Here's how the part is built. I have some questions about the finished solid (model axes, mm). A direction names the side the tool comes from. Round coordinates to 2 decimals unless told otherwise and drop trailing zeros. Write each loop counter-clockwise with the first axis right and the second up, starting at its lowest first coordinate (ties: lowest second). Pieces come first, ordered by that corner, then holes. Notation, with made-up numbers: (17.5, 60) -> (34.5, 60) arc R22 ccw to (34.5, 82) -> close; hole circle Ø2 at (-18.5, 40.25). An arc over 180 degrees is marked (long way). Put each result on its own line as item: value. Start each with the question number.
1) I want a section at A-A, the plane z = -1.75. List the corners of the cut face in (x, y) for me.
2) If I drill on line 1 along Y through (x, z) = (0, -1.95); line 2 along Y through (x, z) = (21, 1.7); line 3 along X through (y, z) = (-15.5, 1.85), over which ranges is the centre line in solid material (lowest first)? Write a range as [from, to].
3) We'd pull the mould along X, two halves only. Please class faces 5 (the flat face through (14.75, 0, 0)), 6 (the cylindrical face through (-18.365, -18.049, 0.042)), 7 (the flat face through (0, 14.75, 0)): released by +X, released by -X, zero draft, split by the parting line, or undercut.
4) Will these pins go through, and if not, where does the flat tip stop? P1, Ø3, axis at y = 18.5, z = 0, coming from the +X side; P2, Ø1.8, axis at y = -19.5, z = -1, coming from the +X side; P3, Ø1.5, axis at x = -12.5, z = -0.5, coming from the -Y side.
5) I want a section at C-C, the plane z = 1.25. List the corners of the cut face in (x, y) for me.
6) Which directions (+Z, -Z, +X, -X, +Y, -Y) give clear straight access to the entire face, cutting with the end or side of a thin tool? Please do faces 1 (the flat face through (-14.75, 0, 0)), 2 (the cylindrical face through (-2.4, -4.5, -1.8)), 3 (the flat face through (4.25, -20, 0)), 4 (the flat face through (-4.25, 20, 0)).
7) I want a section at B-B, the plane y = 17. List the corners of the cut face in (x, z) for me.
8) I want a section at D-D, the plane x = 21.5. List the corners of the cut face in (y, z) for me, then the cut area to 3 significant figures.
from build123d import *

# Parameters (mm, degrees)
BOSS_EXTRUDE1_DEPTH = 3
SKETCH3_R           = 5.1
CUT_EXTRUDE1_DEPTH  = 2.5


with BuildPart() as part:
    # Sketch2 → Boss-Extrude1 (new, symmetric)
    with BuildSketch(Plane.XY):
        with BuildLine():
            Line((-25.396850198, 4.25), (-14.75, 4.25))
            Line((-14.75, 4.25), (-14.75, -4.25))
            Line((-14.75, -4.25), (-25.396850198, -4.25))
            ThreePointArc((-25.396850198, -4.25), (-18.207999616, -18.207999616), (-4.25, -25.396850198))
            Line((-4.25, -25.396850198), (-4.25, -14.75))
            Line((-4.25, -14.75), (4.25, -14.75))
            Line((4.25, -14.75), (4.25, -25.396850198))
            ThreePointArc((4.25, -25.396850198), (18.207999616, -18.207999616), (25.396850198, -4.25))
            Line((25.396850198, -4.25), (14.75, -4.25))
            Line((14.75, -4.25), (14.75, 4.25))
            Line((14.75, 4.25), (25.396850198, 4.25))
            ThreePointArc((25.396850198, 4.25), (18.207999616, 18.207999616), (4.25, 25.396850198))
            Line((4.25, 25.396850198), (4.25, 14.75))
            Line((4.25, 14.75), (-4.25, 14.75))
            Line((-4.25, 14.75), (-4.25, 25.396850198))
            ThreePointArc((-4.25, 25.396850198), (-18.207999616, 18.207999616), (-25.396850198, 4.25))
        make_face()
    extrude(amount=BOSS_EXTRUDE1_DEPTH, both=True)

    # Sketch3 → Cut-Extrude1 (cut)
    with BuildSketch(Plane(origin=(0, 0, -3), x_dir=(-1, 0, 0), z_dir=(0, 0, -1))):
        Circle(SKETCH3_R)
    extrude(amount=-CUT_EXTRUDE1_DEPTH, mode=Mode.SUBTRACT)


solid = part.part
Findings:
1. outline: (-25.4, -4.25) arc R25.75 ccw to (-4.25, -25.4) -> (-4.25, -14.75) -> (4.25, -14.75) -> (4.25, -25.4) arc R25.75 ccw to (25.4, -4.25) -> (14.75, -4.25) -> (14.75, 4.25) -> (25.4, 4.25) arc R25.75 ccw to (4.25, 25.4) -> (4.25, 14.75) -> (-4.25, 14.75) -> (-4.25, 25.4) arc R25.75 ccw to (-25.4, 4.25) -> (-14.75, 4.25) -> (-14.75, -4.25) -> close; hole circle Ø10.2 at (0, 0)
2. line 1: y = [-14.75, -5.1], [5.1, 14.75]
2. line 2: y = [-14.9, -4.25], [4.25, 14.9]
2. line 3: x = [-20.56, -4.25], [4.25, 20.56]
3. face 5: released by +X
3. face 6: released by -X
3. face 7: undercut
4. P1: stops at x = 19.34
4. P2: stops at x = 17.81
4. P3: stops at y = -22.91
5. outline: (-25.4, -4.25) arc R25.75 ccw to (-4.25, -25.4) -> (-4.25, -14.75) -> (4.25, -14.75) -> (4.25, -25.4) arc R25.75 ccw to (25.4, -4.25) -> (14.75, -4.25) -> (14.75, 4.25) -> (25.4, 4.25) arc R25.75 ccw to (4.25, 25.4) -> (4.25, 14.75) -> (-4.25, 14.75) -> (-4.25, 25.4) arc R25.75 ccw to (-25.4, 4.25) -> (-14.75, 4.25) -> (-14.75, -4.25) -> close
6. face 1: +Z, -Z, -X
6. face 2: -Z
6. face 3: +Z, -Z, -Y
6. face 4: +Z, -Z, +Y
7. outline: (-19.34, -3) -> (-4.25, -3) -> (-4.25, 3) -> (-19.34, 3) -> close; (4.25, -3) -> (19.34, -3) -> (19.34, 3) -> (4.25, 3) -> close
8. outline: (-14.17, -3) -> (-4.25, -3) -> (-4.25, 3) -> (-14.17, 3) -> close; (4.25, -3) -> (14.17, -3) -> (14.17, 3) -> (4.25, 3) -> close
8. area: 119 mm2
